Part model, mm, in its own coordinate system. Face numbers are marked on the shaded views. A direction names the side the tool comes from. Give positions to 0.01 mm unless a question says otherwise; leave off trailing zeros. Loops run counter-clockwise (first coordinate to the right, second up) from the corner with the lowest first, then second, coordinate; pieces in that order, holes last. Notation, with made-up numbers: (7.5, 69.25) -> (42.5, 69.25) arc R6 ccw to (42.5, 76.25) -> close; hole circle Ø1 at (85, 7). An arc over 180 degrees is marked (long way). Write item = value, one per line.
from build123d import *

# Parameters (mm, degrees)
SKIZZE1_W                            = 12.5
SKIZZE1_H                            = 5
AUFSATZ_LINEAR_AUSTRAGEN1_DEPTH      = 12
SKIZZE2_W                            = 15
SKIZZE2_H                            = 7.5
AUFSATZ_LINEAR_AUSTRAGEN2_DEPTH      = 21
AUFSATZ_LINEAR_AUSTRAGEN3_DEPTH      = 3.75
AUFSATZ_LINEAR_AUSTRAGEN3_DEPTH_BACK = 3.75
SKIZZE4_R                            = 3.75
AUFSATZ_LINEAR_AUSTRAGEN4_DEPTH      = 13


with BuildPart() as part:
    # Skizze1 → Aufsatz-Linear austragen1 (new body)
    with BuildSketch(Plane.XY):
        Rectangle(SKIZZE1_W, SKIZZE1_H)
    extrude(amount=AUFSATZ_LINEAR_AUSTRAGEN1_DEPTH)

    # Skizze2 → Aufsatz-Linear austragen2 (add)
    with BuildSketch(Plane(origin=(0, 0, 0), x_dir=(-1, 0, 0), z_dir=(0, 0, -1))):
        Rectangle(SKIZZE2_W, SKIZZE2_H)
    extrude(amount=AUFSATZ_LINEAR_AUSTRAGEN2_DEPTH)

    # Skizze3 → Aufsatz-Linear austragen3 (add, two sides)
    with BuildSketch(Plane(origin=(0, 0, 0), x_dir=(1, 0, 0), z_dir=(0, 1, 0))) as aufsatz_linear_austragen3_sk:
        Polygon((-7.5, 21), (-5.75, 26), (-5.75, 32), (5.75, 32), (5.75, 26), (7.5, 21), align=None)
    extrude(amount=AUFSATZ_LINEAR_AUSTRAGEN3_DEPTH)
    extrude(aufsatz_linear_austragen3_sk.sketch, amount=-AUFSATZ_LINEAR_AUSTRAGEN3_DEPTH_BACK)

    # Skizze4 → Aufsatz-Linear austragen4 (add)
    with BuildSketch(Plane(origin=(0, 0, -32), x_dir=(-1, 0, 0), z_dir=(0, 0, -1))):
        Circle(SKIZZE4_R)
    extrude(amount=AUFSATZ_LINEAR_AUSTRAGEN4_DEPTH)


solid = part.part
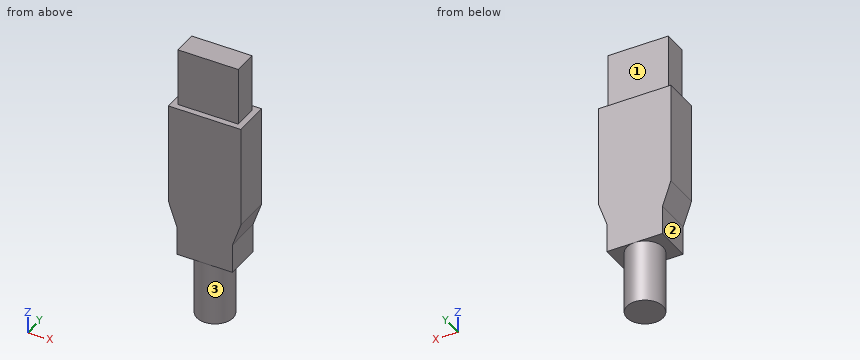
1) Slice it at B-B, the plane x = -4.5. List the corners of the cut face in (y, z).
Resolved:
outline = (-3.75, -32) -> (3.75, -32) -> (3.75, 0) -> (2.5, 0) -> (2.5, 12) -> (-2.5, 12) -> (-2.5, 0) -> (-3.75, 0) -> close
2) Which spindle directions (+Z, -Z, +X, -X, +Y, -Y) get a long thin tool onto all of the face, cutting with end or side? Do the marked faces 1, 2 and 3. Say none if no direction does.
Resolved:
face_1 = +Z, +X, -X, +Y
face_2 = -Z, -X, +Y, -Y
face_3 = -Z
3) Drill centre lines: line 1 along Z through (x, y) = (0, 3); line 2 along X through (y, z) = (1.25, -27); line 3 along Y through (x, z) = (-1.25, 5). Where is each one in solid material? Low to high. Write a range as [from, to].
Resolved:
line_1 = [-45, 0]
line_2 = [-5.75, 5.75]
line_3 = [-2.5, 2.5]
4) Slice it at A-A, the plane y = 0. List the corners of the cut face in (x, z), and give its area (3 significant figures).
Resolved:
outline = (-7.5, -21) -> (-5.75, -26) -> (-5.75, -32) -> (-3.75, -32) -> (-3.75, -45) -> (3.75, -45) -> (3.75, -32) -> (5.75, -32) -> (5.75, -26) -> (7.5, -21) -> (7.5, 0) -> (6.25, 0) -> (6.25, 12) -> (-6.25, 12) -> (-6.25, 0) -> (-7.5, 0) -> close
area = 698 mm²
5) Slice it at D-D, the plane x = 2.25. List the corners of the cut face in (y, z), and give its area (3 significant figures).
Resolved:
outline = (-3.75, -32) -> (-3, -32) -> (-3, -45) -> (3, -45) -> (3, -32) -> (3.75, -32) -> (3.75, 0) -> (2.5, 0) -> (2.5, 12) -> (-2.5, 12) -> (-2.5, 0) -> (-3.75, 0) -> close
area = 378 mm²
6) Slice it at C-C, the plane z = 1.5. List the corners of the cut face in (x, y), and give its area (3 significant figures).
Resolved:
outline = (-6.25, -2.5) -> (6.25, -2.5) -> (6.25, 2.5) -> (-6.25, 2.5) -> close
area = 62.5 mm²
7) Drop flat-ended pins along their axis: P1, Ø2, axis at y = -2, z = 1.5, coming from the +X side; P2, Ø3, axis at y = -1, z = -29, coming from the -X side; P3, Ø5, axis at x = -4, z = -35.5, coming from the -Y side. Give the stop position or say it passes through.
Resolved:
P1 = 6.25
P2 = -5.75
P3 = -3.44
